Design review of the part built by this model. Coordinates are the model's own, in mm. Coordinates: 2 decimals unless noted, no trailing zeros. Loops run counter-clockwise (first coordinate to the right, second up) from the corner with the lowest first, then second, coordinate; pieces in that order, holes last. Notation, with made-up numbers: (22.5, 22) -> (53.5, 22) arc R25 cw to (53.5, 57) -> close; hole circle Ø3 at (65, 5.5). An arc over 180 degrees is marked (long way). Answer in a Markdown table with one row per item.
Autodesk Inventor part; units mm, degrees
ref_plane "Work Plane1" through (0, 485, 0) normal (0, -1, 0) x (1, 0, 0)
ref_plane "YZ Plane" through (0, 0, 0) normal (1, 0, 0) x (0, 1, 0)
ref_plane "XZ Plane" through (0, 0, 0) normal (0, 1, 0) x (-1, 0, 0)
sketch "Sketch1" plane through (0, 0, 0) normal (0, 1, 0) x (-1, 0, 0)
  line L0 (-12, 14) -> (12, 14) construction
  line L1 (14, 12) -> (14, -12) construction
  line L2 (12, -14) -> (-12, -14) construction
  line L3 (-14, -12) -> (-14, 12) construction
  line L4 (-14, 14) -> (14, -14) construction
  line L5 (14, 14) -> (-14, -14) construction
  arc A0 (14, 12) -> (12, 14) centre (12, 12) ccw construction
  arc A1 (12, -14) -> (14, -12) centre (12, -12) ccw construction
  arc A2 (-14, -12) -> (-12, -14) centre (-12, -12) ccw construction
  arc A3 (-12, 14) -> (-14, 12) centre (-12, 12) ccw construction
  line L6 (-12, -15) -> (12, -15)
  arc A4 (12, -15) -> (15, -12) centre (12, -12) ccw
  line L7 (15, -12) -> (15, 12)
  arc A5 (15, 12) -> (12, 15) centre (12, 12) ccw
  line L8 (12, 15) -> (-12, 15)
  arc A6 (-12, 15) -> (-15, 12) centre (-12, 12) ccw
  line L9 (-15, 12) -> (-15, -12)
  arc A7 (-15, -12) -> (-12, -15) centre (-12, -12) ccw
  line L10 (13, -12) -> (13, 12)
  arc A8 (13, 12) -> (12, 13) centre (12, 12) ccw
  line L11 (12, 13) -> (-12, 13)
  arc A9 (-12, 13) -> (-13, 12) centre (-12, 12) ccw
  line L12 (-13, 12) -> (-13, -12)
  arc A10 (-13, -12) -> (-12, -13) centre (-12, -12) ccw
  line L13 (-12, -13) -> (12, -13)
  arc A11 (12, -13) -> (13, -12) centre (12, -12) ccw
  point P0 (0, 0)
  point P1 (0, 0)
  point P2 (0, 0)
  dimension "d10" = 2
  dimension "depth" = 30
  dimension "width" = 30
  dimension "thickness" = 2
extrude "Extrusion1" add sketch "Sketch1" along normal blind 970
ref_plane "Work Plane1" through (0, 485, 0) normal (0, -1, 0) x (1, 0, 0)
sketch "Sketch3" plane through (12, 0, -15) normal (0, 0, -1) x (-1, 0, 0)
  line L0 (12, -397) -> (12, 2382) construction
  circle A0 centre (-3, 1000) radius 985
  point P0 (12, 0)
  dimension "d29" = 1970
  dimension "d31" = 1000
  dimension "d34" = 15
extrude "Extrusion2" cut sketch "Sketch3" against normal through all keep common part
equation "\"d10\" = thickness"
properties part number "podest duzy profil 2" material "Steel"
(1) Take a section at C-C on x = 6. Give the boundary of the cut face in (y, z), and give its area (3 significant figures).
Evaluation:
| item | result |
|---|---|
| outline | (15.04, -15) -> (970, -15) -> (970, -13) -> (15.04, -13) -> close; (15.04, 13) -> (970, 13) -> (970, 15) -> (15.04, 15) -> close |
| area | 3,820 mm² |
(2) To check wall thickness, follow probe 1 along Z at (x, y) = (2, 882); probe 2 along X at (y, z) = (391, 12.5). State the ranges of each line that lie inside material, in increasing order.
Evaluation:
| item | result |
|---|---|
| probe 1 | z = -15 to -13, 13 to 15 |
| probe 2 | x = -14.96 to -12.87, 12.87 to 14.96 |
(3) Take a section at B-B on z = 2. Give the boundary of the cut face in (x, y).
Evaluation:
| item | result |
|---|---|
| outline | (-15, 15.46) arc R985 ccw to (-13, 15.4) -> (-13, 970) -> (-15, 970) -> close; (13, 15) arc R985 ccw to (15, 15) -> (15, 970) -> (13, 970) -> close |
(4) Take a section at A-A on y = 83.5. Give the boundary of the cut face in (x, z).
Evaluation:
| item | result |
|---|---|
| outline | (-15, -12) arc R3 ccw to (-12, -15) -> (12, -15) arc R3 ccw to (15, -12) -> (15, 12) arc R3 ccw to (12, 15) -> (-12, 15) arc R3 ccw to (-15, 12) -> close; hole (-13, -12) arc R1 ccw to (-12, -13) -> (12, -13) arc R1 ccw to (13, -12) -> (13, 12) arc R1 ccw to (12, 13) -> (-12, 13) arc R1 ccw to (-13, 12) -> close |
(5) Draft analysis for pull direction X (two halves, no side actions). For faces 1 (the flat face through (0, 486, 13)), 2 (the flat face through (13, 486, 0)), 3 (the flat face through (-15, 486, 0)), 4 (the flat face through (0, 486, -15)), state which applies: pulls with the +X half, pulls with the -X half, needs draft (parallel to the pull), parting line crosses it, or undercut.
Evaluation:
| item | result |
|---|---|
| face 1 | undercut |
| face 2 | undercut |
| face 3 | pulls with the -X half |
| face 4 | needs draft |
(6) For pin 1 (5 mm diameter, centred on x = 5, z = 10, fed in from +Y), flat-tipped, find the tip position at first contact; note if it passes through.
Evaluation:
| item | result |
|---|---|
| pin 1 | passes through |
